```python
from build123d import *

# Parameters (mm, degrees)
SKETCH1_W           = 40
SKETCH1_H           = 40
BOSS_EXTRUDE1_DEPTH = 40
SKETCH2_W           = 10
SKETCH2_H           = 10
CUT_EXTRUDE1_DEPTH  = 40
CUT_EXTRUDE2_DEPTH  = 40
CUT_EXTRUDE3_DEPTH  = 40
CUT_EXTRUDE4_DEPTH  = 40


with BuildPart() as part:
    # Sketch1 → Boss-Extrude1 (new body)
    with BuildSketch(Plane.XY):
        with Locations((20, 20)):
            Rectangle(SKETCH1_W, SKETCH1_H)
    extrude(amount=BOSS_EXTRUDE1_DEPTH)

    # Sketch2 → Cut-Extrude1 (cut)
    with BuildSketch(Plane.XY.offset(40)):
        with Locations((5, 5)):
            Rectangle(SKETCH2_W, SKETCH2_H)
        with Locations((35, 5)):
            Rectangle(SKETCH2_W, SKETCH2_H)
    extrude(amount=-CUT_EXTRUDE1_DEPTH, mode=Mode.SUBTRACT)

    # Sketch3 → Cut-Extrude2 (cut)
    with BuildSketch(Plane.XY.offset(40)):
        with BuildLine():
            Line((0, 40), (0, 20))
            ThreePointArc((0, 20), (5.857864376, 34.142135624), (20, 40))
            Line((20, 40), (0, 40))
        make_face()
        with BuildLine():
            Line((40, 40), (20, 40))
            ThreePointArc((20, 40), (34.142135624, 34.142135624), (40, 20))
            Line((40, 20), (40, 40))
        make_face()
    extrude(amount=-CUT_EXTRUDE2_DEPTH, mode=Mode.SUBTRACT)

    # Sketch4 → Cut-Extrude3 (cut)
    with BuildSketch(Plane(origin=(0, 0, 0), x_dir=(1, 0, 0), z_dir=(0, 1, 0))):
        with BuildLine():
            Line((0, 0), (0, -20))
            ThreePointArc((0, -20), (5.857864376, -5.857864376), (20, 0))
            Line((20, 0), (0, 0))
        make_face()
        with BuildLine():
            Line((40, 0), (20, 0))
            ThreePointArc((20, 0), (34.142135624, -5.857864376), (40, -20))
            Line((40, -20), (40, 0))
        make_face()
    extrude(amount=CUT_EXTRUDE3_DEPTH, mode=Mode.SUBTRACT)

    # Sketch5 → Cut-Extrude4 (cut)
    with BuildSketch(Plane(origin=(0, 0, 0), x_dir=(0, 0, -1), z_dir=(1, 0, 0))):
        Polygon((0, 40), (-20, 20), (-40, 20), (-40, 40), align=None)
    extrude(amount=CUT_EXTRUDE4_DEPTH, mode=Mode.SUBTRACT)


solid = part.part
```
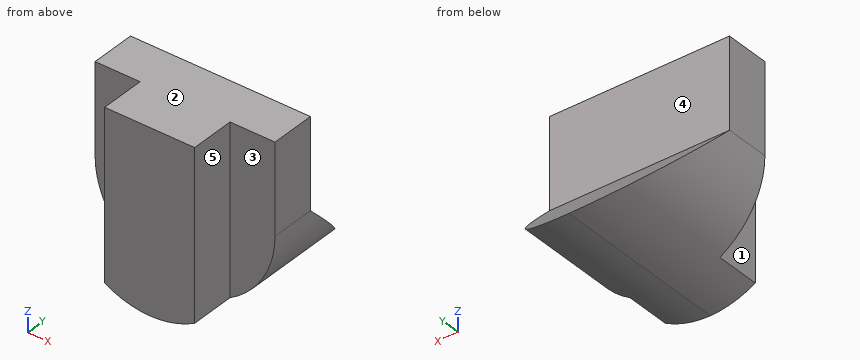
CAD build for the part. Positions are in the model's coordinates, mm. Face numbers are marked on the shaded views. A direction names the side the tool comes from. Coordinates: 2 decimals unless noted, no trailing zeros. Loops run counter-clockwise (first coordinate to the right, second up) from the corner with the lowest first, then second, coordinate; pieces in that order, holes last. Notation, with made-up numbers: (-29, 47) - (-15, 47) arc R20 cw to (-15, 68) - close; hole circle Ø2 at (-17.75, 39). An arc over 180 degrees is marked (long way). Use CSV: the item, a comma, the result in double quotes. Start each with the question number.
Q1. Cut at B-B, the plane y = 6.5. List the corners of the cut face in (x, z).
Q2. Cut at A-A, the plane z = 4. List the corners of the cut face in (x, y), then the cut area to 3 significant figures.
Q3. Probe probe 1 along Y at (x, z) = (26.5, 36.5); probe 2 along X at (y, z) = (2, 10); probe 3 along Y at (x, z) = (37.5, 21.5). List the from-to ranges inside material, lowest first. Write a range as from..to.
Q4. 3-axis set-ups, long thin cutter, end or side, ignore diameter. For the marked faces 1 and 2: which of +Z, -Z, +X, -X, +Y, -Y reach the whole face in a straight line?
Q5. Drop flat-ended pins along their axis: P1, Ø3, axis at x = 15.5, y = 19.5, coming from the -Z side; P2, Ø8, axis at x = 37, z = 26, coming from the -Y side; P3, Ø5, axis at y = 4, z = 12.5, coming from the +X side; P4, Ø11, axis at x = 7, z = 14, coming from the -Y side. Give the stop position or say it passes through.
Q6. Cut at D-D, the plane z = 26. List the corners of the cut face in (x, y), then the cut area to 3 significant figures.
Q7. Cut at C-C, the plane x = 32. List the corners of the cut face in (y, z).
Q8. Two-plate mould, pull along Y, no slides. Class the marked faces 3, 4 and 5: +Y half, -Y half, draft (parallel to the pull), parting line (faces both ways), or undercut.
Here are the results:
1,outline,"(10, 2.68) arc R20 ccw to (30, 2.68) - (30, 40) - (10, 40) - close"
2,outline,"(8, 10) - (10, 10) - (10, 0) - (30, 0) - (30, 10) - (32, 10) - (32, 36) - (8, 36) - close"
2,area,"824 mm2"
3,probe 1,"0..20"
3,probe 2,"10..30"
3,probe 3,"10..20"
4,face 1,"+Z, -Z, -X, -Y"
4,face 2,"+Z, +X, -X, +Y, -Y"
5,P1,"z = 0.23"
5,P2,"y = 10"
5,P3,"x = 30"
5,P4,"y = 0"
6,outline,"(0, 10) - (10, 10) - (10, 0) - (30, 0) - (30, 10) - (40, 10) - (40, 20) - (0, 20) - close"
6,area,"600 mm2"
7,outline,"(10, 4) - (36, 4) - (20, 20) - (20, 40) - (10, 40) - close"
8,face 3,"-Y half"
8,face 4,"+Y half"
8,face 5,"draft"
